Here's the drawing with two shaded views (mm, measured from the low corner). I have some questions. A direction names the side the tool comes from. Give positions to 0.01 mm unless a question says otherwise; leave off trailing zeros. Write each loop counter-clockwise with the first axis right and the second up, starting at its lowest first coordinate (ties: lowest second). Pieces come first, ordered by that corner, then holes. Notation, with made-up numbers: (-13, 58) -> (37, 58) arc R7 cw to (37, 62) -> close; hole circle Ø6 at (-36.5, 45.25). An arc over 180 degrees is marked (long way). One line per question, with ' | ' between items.
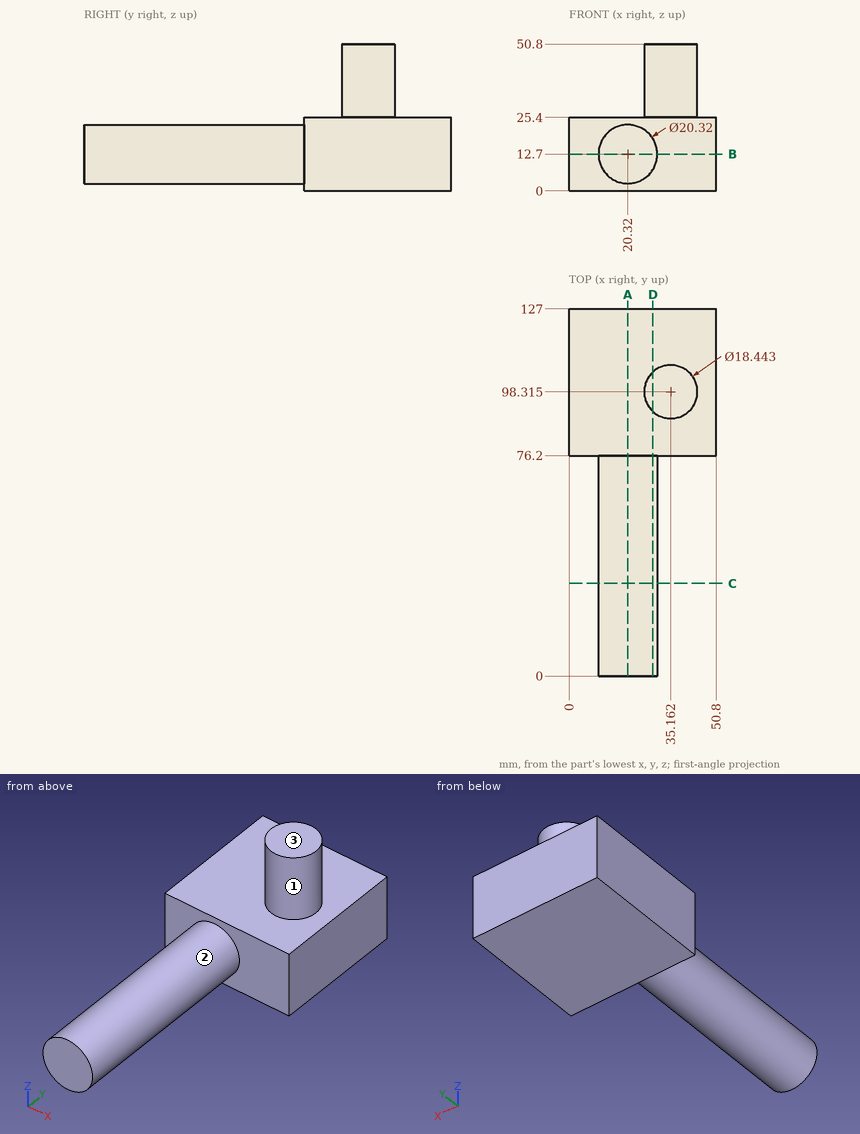
Q1. Imagine slicing it at A-A on x = 20.32. Please give me the cut outline in (y, z).
Answer below:
outline: (0, 2.54) -> (76.2, 2.54) -> (76.2, 0) -> (127, 0) -> (127, 25.4) -> (76.2, 25.4) -> (76.2, 22.86) -> (0, 22.86) -> close
Q2. Imagine slicing it at C-C on y = 32. Please give me the cut outline in (x, z), and give its area (3 significant figures).
Answer below:
outline: circle Ø20.32 at (20.32, 12.7) | area: 324 mm^2
Q3. On a 3-axis mill with a long thin cutter (end or side, diameter ignored), from which of +Z, -Z, +X, -X, +Y, -Y can I reach the whole of each face in a straight line? I mean the marked faces 1, 2 and 3. Say none if no direction works.
Answer below:
face 1: +Z | face 2: -Y | face 3: +Z, +X, -X, +Y, -Y
Q4. Imagine slicing it at D-D on x = 29. Please give me the cut outline in (y, z) (1 decimal).
Answer below:
outline: (0, 7.4) -> (76.2, 7.4) -> (76.2, 0) -> (127, 0) -> (127, 25.4) -> (105.2, 25.4) -> (105.2, 50.8) -> (91.5, 50.8) -> (91.5, 25.4) -> (76.2, 25.4) -> (76.2, 18) -> (0, 18) -> close
Q5. Will these pins go through, and if not, where does the flat tip stop? pin 1 (3 mm diameter, centred on x = 25, y = 82, fed in from -Z); pin 2 (5 mm diameter, centred on y = 106, z = 39, fed in from -X) (1 decimal); pin 3 (5 mm diameter, centred on y = 96, z = 31.5, fed in from +X); pin 4 (1.5 mm diameter, centred on x = 6, z = 14.5, fed in from -Y).
Answer below:
pin 1: stops at z = 0 | pin 2: stops at x = 27.5 | pin 3: stops at x = 44.38 | pin 4: stops at y = 76.2
Q6. If I drill on line 1 along Z through (x, y) = (21, 22.5); line 2 along Z through (x, y) = (10.5, 119.5); line 3 along Y through (x, z) = (46, 20), over which ranges is the centre line in solid material (lowest first)?
Answer below:
line 1: z = 2.56 to 22.84 | line 2: z = 0 to 25.4 | line 3: y = 76.2 to 127
Q7. Imagine slicing it at B-B on z = 12.7. Please give me the cut outline in (x, y), and give its area (3 significant figures).
Answer below:
outline: (0, 76.2) -> (10.16, 76.2) -> (10.16, 0) -> (30.48, 0) -> (30.48, 76.2) -> (50.8, 76.2) -> (50.8, 127) -> (0, 127) -> close | area: 4,130 mm^2
